The listing builds one solid part. Answer for the finished solid, in the listing's coordinates (mm). A direction names the side the tool comes from. Round coordinates to 2 decimals unless told otherwise and drop trailing zeros. Write each loop counter-clockwise with the first axis right and the second up, starting at its lowest first coordinate (ties: lowest second). Pieces come first, ordered by that corner, then holes.
Autodesk Inventor part; units mm, degrees
ref_plane "YZ Plane" through (0, 0, 0) normal (1, 0, 0) x (0, 1, 0)
ref_plane "XZ Plane" through (0, 0, 0) normal (0, 1, 0) x (-1, 0, 0)
ref_plane "XY Plane" through (0, 0, 0) normal (0, 0, 1) x (1, 0, 0)
sketch "Sketch1" plane through (0, 0, 0) normal (0, 1, 0) x (-1, 0, 0)
  line L0 (0, 0) -> (16, 0)
  line L1 (16, 0) -> (16, -5)
  line L2 (16, -5) -> (12, -5)
  line L3 (12, -5) -> (12, -10)
  line L4 (12, -10) -> (22, -10)
  line L5 (22, -10) -> (22, 5)
  line L6 (22, 5) -> (-4, 5)
  line L7 (0, 0) -> (0, -5)
  line L8 (0, -5) -> (4, -5)
  line L9 (4, -5) -> (4, -10)
  line L10 (4, -10) -> (-6, -10)
  line L11 (-6, -10) -> (-6, 5)
  line L12 (-6, 5) -> (-4, 5)
  dimension "d0" = 16
  dimension "d1" = 5
  dimension "d2" = 4
  dimension "d3" = 5
  dimension "d4" = 10
  dimension "d5" = 15
  dimension "d6" = 26
  dimension "d11" = 5
  dimension "d12" = 4
  dimension "d13" = 5
  dimension "d14" = 10
  dimension "d15" = 15
extrude "Extrusion1" add sketch "Sketch1" along normal blind 500
sketch "Sketch2" plane through (6, 0, 5) normal (1, 0, 0) x (0, 0, -1)
  line L0 (0, 0) -> (0, 500)
  line L1 (0, 0) -> (0, 80)
  line L2 (0, 80) -> (15, 80)
  line L3 (15, 0) -> (15, 500)
  line L4 (15, 80) -> (35, 80)
  line L5 (35, 80) -> (35, 110)
  line L6 (35, 110) -> (-20, 110)
  line L7 (-20, 110) -> (-20, 50)
  line L8 (-20, 50) -> (35, 50)
  line L9 (35, 50) -> (35, 80)
  line L10 (-20, 110) -> (-10, 110)
  line L11 (-10, 110) -> (-10, 90)
  line L12 (-10, 90) -> (-10, 70)
  line L13 (-10, 70) -> (25, 70)
  line L14 (25, 70) -> (25, 90)
  line L15 (-10, 95) -> (-15.9639, 95)
  line L16 (-10, 65) -> (-17.5959, 65)
  circle A0 centre (25, 95) radius 5
  circle A1 centre (-10, 95) radius 5
  circle A2 centre (25, 65) radius 5
  circle A3 centre (-10, 65) radius 5
  point P0 (5, 0)
  dimension "d18" = 80
  dimension "d19" = 15
  dimension "d20" = 20
  dimension "d21" = 30
  dimension "d22" = 55
  dimension "d23" = 60
  dimension "d24" = 10
  dimension "d25" = 20
  dimension "d26" = 20
  dimension "d27" = 35
  dimension "d28" = 20
  dimension "d33" = 10
  dimension "d34" = 10
  dimension "d35" = 10
  dimension "d36" = 10
extrude "Extrusion2" add sketch "Sketch2" along normal blind 3 contours L8 L7 L6 L11 A1 L12 L13 L0 | L0 L13 L3 L8 | L13 L12 A1 L11 L6 L0 | L0 L2 L3 L13 | L3 L13 L14 L4 L9 L8 | L0 L6 L3 L2 | L3 L4 L14 L13 | L3 L6 L5 L4
sketch "Sketch3" plane through (6, 0, 5) normal (-1, 0, 0) x (0, 0, 1)
  line L0 (20, 50) -> (-35, 50)
  line L1 (-35, 50) -> (-35, 110)
  line L2 (-35, 50) -> (-35, 110)
  line L3 (-35, 110) -> (20, 110)
  line L4 (-35, 110) -> (20, 110)
  line L5 (20, 110) -> (20, 50)
  line L6 (20, 110) -> (20, 50)
  line L7 (20, 50) -> (-35, 50)
  point P0 (-5, 0)
extrude "Extrusion3" add sketch "Sketch3" against normal blind 3
sketch "Sketch4" plane through (6, 0, 5) normal (-1, 0, 0) x (0, 0, 1)
  line L0 (0, 50) -> (0, 110)
  line L1 (0, 50) -> (9, 50)
  line L2 (20, 50) -> (-35, 50)
  line L3 (9, 50) -> (9, 110)
  line L4 (-35, 110) -> (20, 110)
  line L5 (9, 110) -> (23.2747, 110)
  line L6 (-35, 110) -> (-15, 110)
  line L7 (23.2747, 110) -> (23.2747, 50)
  line L8 (23.2747, 50) -> (9, 50)
  line L9 (-15, 50) -> (-35, 50)
  line L10 (-15, 50) -> (-24, 50)
  line L11 (-24, 50) -> (-24, 110)
  line L12 (-24, 110) -> (-51.0156, 108.7427)
  line L13 (-51.0156, 108.7427) -> (-51.1782, 112.2347)
  line L14 (-51.1782, 112.2347) -> (-24, 110)
  line L15 (-51.0156, 108.7427) -> (-55.6093, 34.9275)
  line L16 (-55.6093, 34.9275) -> (-24, 50)
  point P0 (-5, 0)
  dimension "d41" = 9
  dimension "d42" = 9
extrude "Extrusion4" cut sketch "Sketch4" against normal blind 3 contours L3 L4 L5 L7 L8 L2 | L16 L15 L12 L11 | L12 L13 L14
sketch "Sketch5" plane through (6, 0, 5) normal (-1, 0, 0) x (0, 0, 1)
  line L0 (-15, 50) -> (-24, 50)
  line L1 (-24, 50) -> (-19.5, 50)
  circle A0 centre (-19.5, 95) radius 2.5
  circle A1 centre (-19.5, 80) radius 2.5
  circle A2 centre (-19.5, 65) radius 2.5
  line L2 (9, 50) -> (0, 50)
  line L3 (9, 50) -> (4.5, 50)
  circle A3 centre (4.5, 95) radius 2.5
  circle A4 centre (4.5, 80) radius 2.5
  circle A5 centre (4.5, 65) radius 2.5
  point P0 (-5, 0)
  dimension "d48" = 5
  dimension "d49" = 5
  dimension "d50" = 5
  dimension "d51" = 4.5
  dimension "d52" = 5
  dimension "d53" = 5
  dimension "d54" = 5
extrude "Extrusion5" cut sketch "Sketch5" against normal blind 3
thicken "Thicken1" operation add thickness 200 both sides no extend neighbours yes toward (0, 1, 0) faces at (-5.3333, 500, 3.3333)
properties part number "Guia"
1. Given pin 1 (12 mm diameter, centred on x = 0.5, y = 588, fed in from -Z); pin 2 (3 mm diameter, centred on y = 80, z = 9.5, fed in from +X); pin 3 (6 mm diameter, centred on y = 145.5, z = -0.5, fed in from +X); pin 4 (1.2 mm diameter, centred on x = -2, y = 344.5, fed in from +Z), each flat-ended and moving along its own axis, determine where each tip first touches the part or whether it passes through.
Geometry says:
pin 1: stops at z = -10
pin 2: passes through
pin 3: stops at x = 6
pin 4: stops at z = 5
2. Section A-A on y = 185 is taken. Determine the outline of the cut face in (x, z), plus the area to 3 significant figures.
Geometry says:
outline: (-22, -10) - (-12, -10) - (-12, -5) - (-16, -5) - (-16, 0) - (0, 0) - (0, -5) - (-4, -5) - (-4, -10) - (6, -10) - (6, 5) - (-22, 5) - close
area: 300 mm2
3. For a pull along X with two mould halves and no side action, classify faces 4 (the face through (-8, 345, 0)), 5 (the face through (-22, 345, -3)), 6 (the face through (9, 80, -2)), 7 (the face through (-8, 345, 5)) as released by +X, released by -X, zero draft, split by the parting line, or undercut.
Geometry says:
face 4: undercut
face 5: released by -X
face 6: released by +X
face 7: zero draft
4. A tool of negligible diameter and unlimited length cuts with its end or side. For faces 1 (the face through (6, 401, -3)), 2 (the face through (-8, 0, 1)), 3 (the face through (6, 25, -3)), from which of +Z, -Z, +X, -X, +Y, -Y can it reach the whole face along a straight path? Write none if from no direction.
Geometry says:
face 1: +Z, -Z, +X, +Y
face 2: +Z, -Z, +X, -X, -Y
face 3: +Z, -Z, +X, -Y
5. Straight lines are drawn through the part: line 1 along Y through (x, z) = (7, 9); line 2 along Z through (x, y) = (-2.5, 462); line 3 along X through (y, z) = (606, -4.5). For each, find the intervals that lie inside material, in ascending order.
Geometry says:
line 1: y = 50 to 62.55, 67.45 to 77.55, 82.45 to 92.55, 97.45 to 110
line 2: z = -10 to -5, 0 to 5
line 3: x = -22 to -16, 0 to 6
